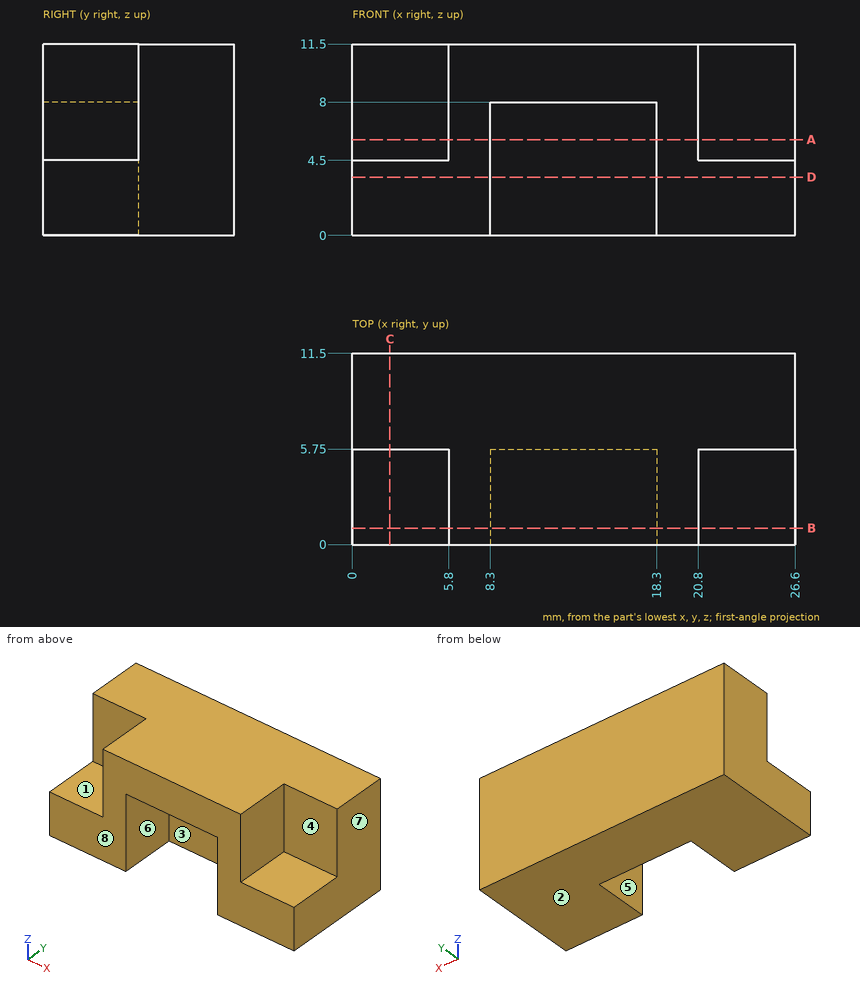
Can you work these out from the drawing? Everything is in mm from the part's minimum corner. A direction names the side the tool comes from. Coordinates: 2 decimals unless noted, no trailing zeros. Loops run counter-clockwise (first coordinate to the right, second up) from the corner with the lowest first, then second, coordinate; pieces in that order, holes last. Notation, with made-up numbers: (88, 51) - (102, 51) arc R13 cw to (102, 56) - close; hole circle Ø11 at (-4.5, 46). An arc over 180 degrees is marked (long way). Use a Markdown table: item, result.
Item 1: We'd pull the mould along X, two halves only. Please class the marked faces 5, 6, 7 and 8: released by +X, released by -X, zero draft, split by the parting line, or undercut.
Numbers:
| item | result |
|---|---|
| face 5 | undercut |
| face 6 | undercut |
| face 7 | released by +X |
| face 8 | zero draft |
Item 2: I want a section at C-C on x = 2.25. Please give me the cut outline in (y, z).
Numbers:
| item | result |
|---|---|
| outline | (0, 0) - (11.5, 0) - (11.5, 11.5) - (5.75, 11.5) - (5.75, 4.5) - (0, 4.5) - close |
Item 3: If I drill on probe 1 along X at (y, z) = (1.5, 4.25); probe 2 along Y at (x, z) = (14.25, 5); probe 3 along X at (y, z) = (1.25, 7.5), over which ranges is the centre line in solid material (lowest first)? Write a range as from..to.
Numbers:
| item | result |
|---|---|
| probe 1 | x = 0..8.3, 18.3..26.6 |
| probe 2 | y = 5.75..11.5 |
| probe 3 | x = 5.8..8.3, 18.3..20.8 |
Item 4: I want a section at A-A on z = 5.75. Please give me the cut outline in (x, y), and give its area (3 significant figures).
Numbers:
| item | result |
|---|---|
| outline | (0, 5.75) - (5.8, 5.75) - (5.8, 0) - (8.3, 0) - (8.3, 5.75) - (18.3, 5.75) - (18.3, 0) - (20.8, 0) - (20.8, 5.75) - (26.6, 5.75) - (26.6, 11.5) - (0, 11.5) - close |
| area | 182 mm2 |
Item 5: For the marked faces 1, 2, 3 and 4, which set-ups out of +Z, -Z, +X, -X, +Y, -Y let a thin tool reach every point of the face, with its end or its side?
Numbers:
| item | result |
|---|---|
| face 1 | +Z, -X, -Y |
| face 2 | -Z, +X, -X, +Y, -Y |
| face 3 | -Z, -Y |
| face 4 | +Z, +X, -Y |
Item 6: I want a section at D-D on z = 3.5. Please give me the cut outline in (x, y), and give its area (3 significant figures).
Numbers:
| item | result |
|---|---|
| outline | (0, 0) - (8.3, 0) - (8.3, 5.75) - (18.3, 5.75) - (18.3, 0) - (26.6, 0) - (26.6, 11.5) - (0, 11.5) - close |
| area | 248 mm2 |
Item 7: I want a section at B-B on y = 1. Please give me the cut outline in (x, z), and give its area (3 significant figures).
Numbers:
| item | result |
|---|---|
| outline | (0, 0) - (8.3, 0) - (8.3, 8) - (18.3, 8) - (18.3, 0) - (26.6, 0) - (26.6, 4.5) - (20.8, 4.5) - (20.8, 11.5) - (5.8, 11.5) - (5.8, 4.5) - (0, 4.5) - close |
| area | 145 mm2 |
Item 8: Will these pins go through, and if not, where does the flat tip stop? pin 1 (1.7 mm diameter, centred on y = 2.5, z = 8, fed in from +X); pin 2 (4 mm diameter, centred on x = 11, z = 2.5, fed in from -Y); pin 3 (3 mm diameter, centred on x = 15, y = 4, fed in from -Z).
Numbers:
| item | result |
|---|---|
| pin 1 | stops at x = 20.8 |
| pin 2 | stops at y = 5.75 |
| pin 3 | stops at z = 8 |
